from build123d import *

# Parameters (mm, degrees)
BOSS_EXTRUDE1_DEPTH = 1.5
SKETCH2_W           = 3
SKETCH2_H           = 1.750926398
BOSS_EXTRUDE2_DEPTH = 5
SKETCH3_W           = 20
SKETCH3_H           = 3
BOSS_EXTRUDE3_DEPTH = 25
CUT_EXTRUDE1_DEPTH  = 5
CUT_EXTRUDE2_DEPTH  = 10
BOSS_EXTRUDE4_DEPTH = 3


with BuildPart() as part:
    # Sketch1 → Boss-Extrude1 (new body)
    with BuildSketch(Plane.XY):
        Polygon((3, 46), (11.5, 46), (11.5, 49), (-8.5, 49), (-8.5, 46), (0, 46), (0, 0), (3, 0), align=None)
    extrude(amount=BOSS_EXTRUDE1_DEPTH)

    # Sketch2 → Boss-Extrude2 (add)
    with BuildSketch(Plane.XY.offset(1.5)):
        with Locations((1.5, 0.875463199)):
            Rectangle(SKETCH2_W, SKETCH2_H)
    extrude(amount=BOSS_EXTRUDE2_DEPTH)

    # Sketch3 → Boss-Extrude3 (add)
    with BuildSketch(Plane.XY.offset(1.5)):
        with Locations((1.5, 47.5)):
            Rectangle(SKETCH3_W, SKETCH3_H)
    extrude(amount=BOSS_EXTRUDE3_DEPTH)

    # Sketch4 → Cut-Extrude1 (cut)
    with BuildSketch(Plane.XZ):
        Polygon((1.5, 6.5), (0, 3.25), (-2.721053337, 3.25), (-2.721053337, 9.447530039), (6.003312616, 9.447530039), (5.654337978, 3.25), (3, 3.25), align=None)
    extrude(amount=-CUT_EXTRUDE1_DEPTH, mode=Mode.SUBTRACT)

    # Sketch5 → Cut-Extrude2 (cut)
    with BuildSketch(Plane.XZ.offset(-46)):
        with BuildLine():
            Line((-4, 8), (-4, 3))
            ThreePointArc((-4, 3), (-5.5, 1.5), (-7, 3))
            Line((-7, 3), (-7, 8))
            ThreePointArc((-7, 8), (-5.5, 9.5), (-4, 8))
        make_face()
        with BuildLine():
            Line((10, 8), (10, 3))
            ThreePointArc((10, 3), (8.5, 1.5), (7, 3))
            Line((7, 3), (7, 8))
            ThreePointArc((7, 8), (8.5, 9.5), (10, 8))
        make_face()
        with BuildLine():
            Line((10, 23), (10, 18))
            ThreePointArc((10, 18), (8.5, 16.5), (7, 18))
            Line((7, 18), (7, 23))
            ThreePointArc((7, 23), (8.5, 24.5), (10, 23))
        make_face()
        with BuildLine():
            Line((-4, 23), (-4, 18))
            ThreePointArc((-4, 18), (-5.5, 16.5), (-7, 18))
            Line((-7, 18), (-7, 23))
            ThreePointArc((-7, 23), (-5.5, 24.5), (-4, 23))
        make_face()
    extrude(amount=-CUT_EXTRUDE2_DEPTH, mode=Mode.SUBTRACT)

    # Sketch6 → Boss-Extrude4 (add)
    with BuildSketch(Plane.ZY):
        Polygon((1.5, 46), (16.5, 46), (1.5, 36), align=None)
    extrude(amount=-BOSS_EXTRUDE4_DEPTH)


solid = part.part
CAD build for the part. Positions are in the model's coordinates, mm. A direction names the side the tool comes from. Round coordinates to 2 decimals unless told otherwise and drop trailing zeros. Loops run counter-clockwise (first coordinate to the right, second up) from the corner with the lowest first, then second, coordinate; pieces in that order, holes last.
(1) Cut at B-B (z = 22). Give the cut face in (x, y), plus the area to 3 significant figures.
(2) Which spindle directions (+Z, -Z, +X, -X, +Y, -Y) get a long thin tool onto all of the face, cutting with end or side? Do faces 1 (the flat face through (1, 41, 9)), 2 (the flat face through (3, 35, 1)), 3 (the cylindrical face through (8.5, 47.5, 9.5)). Say none if no direction does.
(3) Wall check: line 1 along X through (y, z) = (44.5, 13); line 2 along Y through (x, z) = (-3, 4.25); line 3 along Y through (x, z) = (2.5, 10.75). Give the ranges that are in metal, low to high.
(4) Cut at C-C (y = 45). Give the cut face in (x, z), plus the area to 3 significant figures.
(5) Drop flat-ended pins along their axis: pin 1 (5 mm diameter, centred on y = 31.5, z = 6, fed in from -X); pin 2 (2.5 mm diameter, centred on x = 1, y = 19.5, fed in from +Z); pin 3 (10 mm diameter, centred on x = 0, y = 5, fed in from +Z). Give the stop position or say it passes through.
(6) Cut at D-D (z = 2). Give the cut face in (x, y).
(7) Two-plate mould, pull along X, no slides. Class faces 4 (the flat face through (1, 49, 13)), 5 (the flat face through (0.76, 0.86, 4.9)), 6 (the flat face through (10, 47, 6)): +X half, -X half, draft (parallel to the pull), parting line (faces both ways), or undercut.
(8) Cut at A-A (x = 8.5). Give the cut face in (y, z), plus the area to 3 significant figures.
Findings below:
1. outline: (-8.5, 46) - (-7, 46) - (-7, 49) - (-8.5, 49) - close; (-4, 46) - (7, 46) - (7, 49) - (-4, 49) - close; (10, 46) - (11.5, 46) - (11.5, 49) - (10, 49) - close
1. area: 42.0 mm2
2. face 1: +Z, +X, -X
2. face 2: +Z, -Z, +X, -Y
2. face 3: +Y, -Y
3. line 1: x = 0 to 3
3. line 2: y = 46 to 49
3. line 3: y = 42.17 to 49
4. outline: (0, 0) - (3, 0) - (3, 15) - (0, 15) - close
4. area: 45.0 mm2
5. pin 1: passes through
5. pin 2: stops at z = 1.5
5. pin 3: stops at z = 6.5
6. outline: (-8.5, 46) - (-6.62, 46) - (-6.62, 49) - (-8.5, 49) - close; (-4.38, 46) - (0, 46) - (0, 36.33) - (3, 36.33) - (3, 46) - (7.38, 46) - (7.38, 49) - (-4.38, 49) - close; (0, 0) - (3, 0) - (3, 1.75) - (0, 1.75) - close; (9.62, 46) - (11.5, 46) - (11.5, 49) - (9.62, 49) - close
7. face 4: draft
7. face 5: -X half
7. face 6: undercut
8. outline: (46, 0) - (49, 0) - (49, 1.5) - (46, 1.5) - close; (46, 9.5) - (49, 9.5) - (49, 16.5) - (46, 16.5) - close; (46, 24.5) - (49, 24.5) - (49, 26.5) - (46, 26.5) - close
8. area: 31.5 mm2
